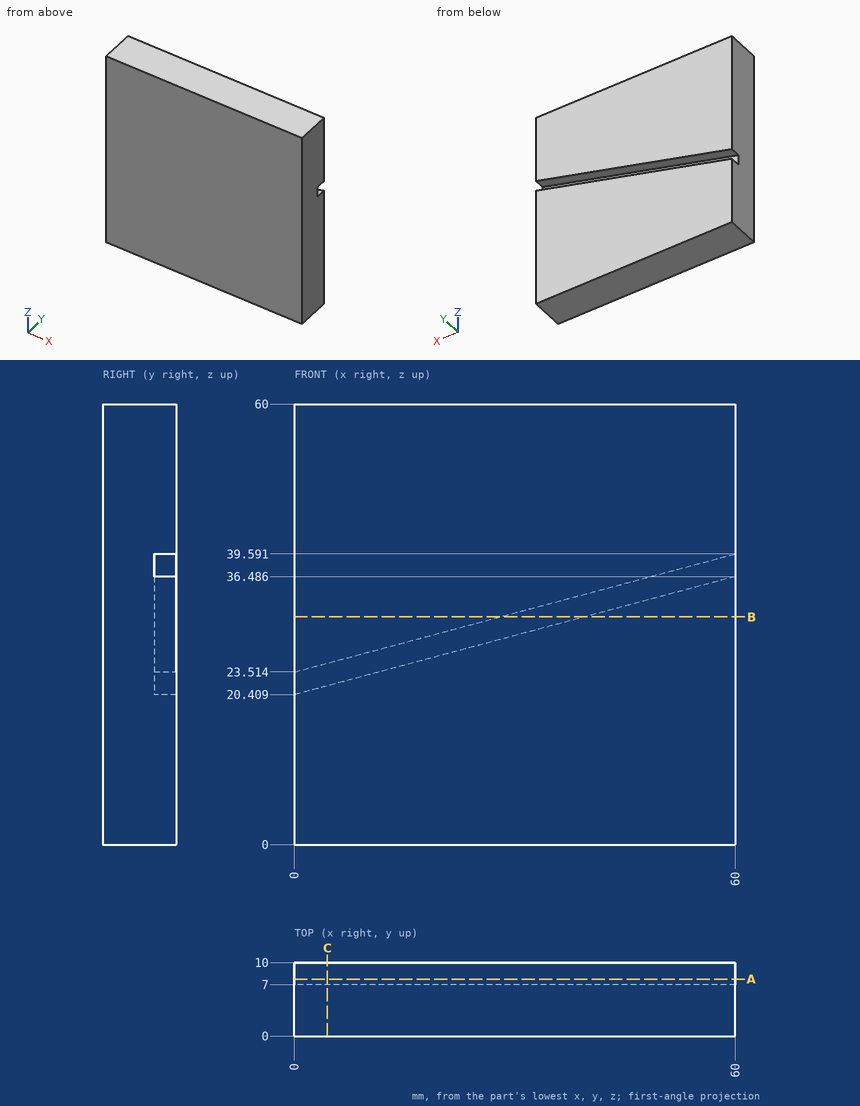
Part print with two shaded views. Sizes in mm from the minimum x, y, z corner. Round coordinates to 2 decimals unless told otherwise and drop trailing zeros. Order: outer loops, then holes, each group sorted by start corner. A loop starts at its lowest first (then second) coordinate and runs counter-clockwise, first axis right, second up. Notation, with made-up numbers: M 43,47 L 96,47 A29 ccw 96,70 Z; hole C -30,-29.5 d11. An arc over 180 degrees is marked long. Answer in a Markdown table with one row per item. Add a question column.
Q1. Cut at C-C on x = 4.5. Give the cut face in (y, z) (1 decimal).
Q2. Wall check: L1, parallel to Z at x = 56.5, y = 8.5; L2, parallel to Z at x = 39.5, y = 9.5; L3, parallel to Y at x = 25.5, z = 28. Give the ranges that are in metal, low to high. Write a range as from..to.
Q3. Cut at A-A on y = 7.75. Give the cut face in (x, z) (1 decimal), and give its area (3 significant figures).
Q4. Cut at B-B on z = 31. Give the cut face in (x, y).
Established:
| question | item | result |
|---|---|---|
| 1 | outline | M 0,0 L 10,0 L 10,21.6 L 7,21.6 L 7,24.7 L 10,24.7 L 10,60 L 0,60 Z |
| 2 | L1 | z = 0..35.55, 38.65..60 |
| 2 | L2 | z = 0..30.99, 34.1..60 |
| 2 | L3 | y = 0..7 |
| 3 | outline | M 0,0 L 60,0 L 60,36.5 L 0,20.4 Z; M 0,23.5 L 60,39.6 L 60,60 L 0,60 Z |
| 3 | area | 3,410 mm2 |
| 4 | outline | M 0,0 L 60,0 L 60,10 L 39.53,10 L 39.53,7 L 27.94,7 L 27.94,10 L 0,10 Z |
